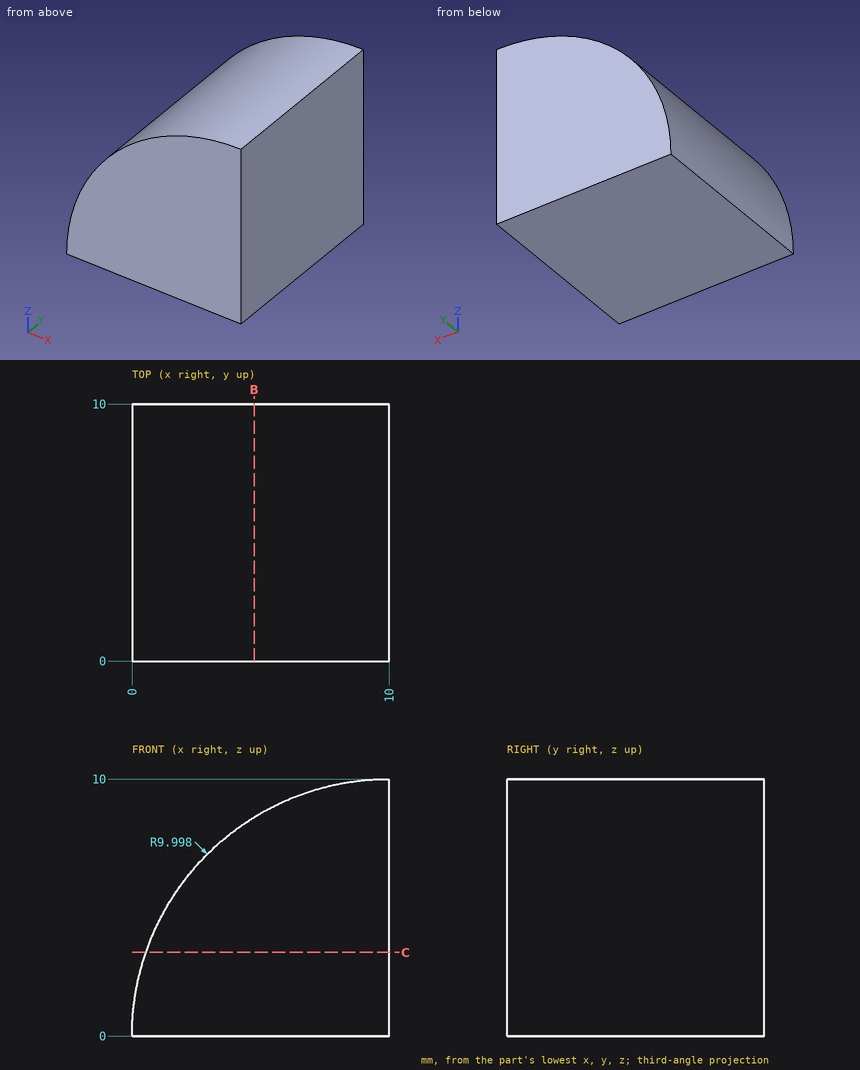
Here's the drawing with two shaded views (mm, measured from the low corner). I have some questions. Coordinates: 2 decimals unless noted, no trailing zeros. Write each loop counter-clockwise with the first axis right and the second up, starting at its lowest first coordinate (ties: lowest second). Pieces come first, ordered by that corner, then holes. Notation, with made-up numbers: M -19.75,8 L 25.25,8 A17 ccw 25.25,19 Z; hole C 29,80 d8. An arc over 180 degrees is marked long. Use one line per item in the form item = value.
Q1. If we section it at C-C (z = 3.25): Write out the boundary of the cut face in (x, y), then the cut area to 3 significant figures.
Model answer:
outline = M 0.54,0 L 10,0 L 10,10 L 0.54,10 Z
area = 94.6 mm^2
Q2. For P1, Ø5, axis at x = 3, y = 5, coming from the +Z side; P2, Ø1.5, axis at x = 5.5, y = 6, coming from the +Z side; P3, Ø1.5, axis at x = 4, y = 1.5, coming from the +Z side, each with a flat end and sliding along its axis, tell me the tip position at first contact or that it passes through.
Model answer:
P1 = 8.93
P2 = 9.27
P3 = 8.51
Q3. I need wall thicknesses on line 1 along X through (y, z) = (5, 4.75); line 2 along X through (y, z) = (8, 8.25); line 3 along Z through (x, y) = (6, 1.75). Which ranges of each line are inside material? Lowest first, please. Write a range as from..to.
Model answer:
line_1 = 1.2..10
line_2 = 4.35..10
line_3 = 0..9.17
Q4. If we section it at B-B (x = 4.75): Write out the boundary of the cut face in (y, z).
Model answer:
outline = M 0,0 L 10,0 L 10,8.51 L 0,8.51 Z
